Source: three-view drawing plus pictorial views. Frame: mm from the lowest corner of the part. Give positions to 0.01 mm unless a question says otherwise; leave off trailing zeros. Loops run counter-clockwise (first coordinate to the right, second up) from the corner with the lowest first, then second, coordinate; pieces in that order, holes last. Notation, with made-up numbers: M -15.75,61.5 L -1.75,61.5 A11 ccw -1.75,82.5 Z; hole C 57.25,-16.5 d9. An arc over 180 degrees is marked long. Answer as a JSON object with one key per item and string values. Group by question number.
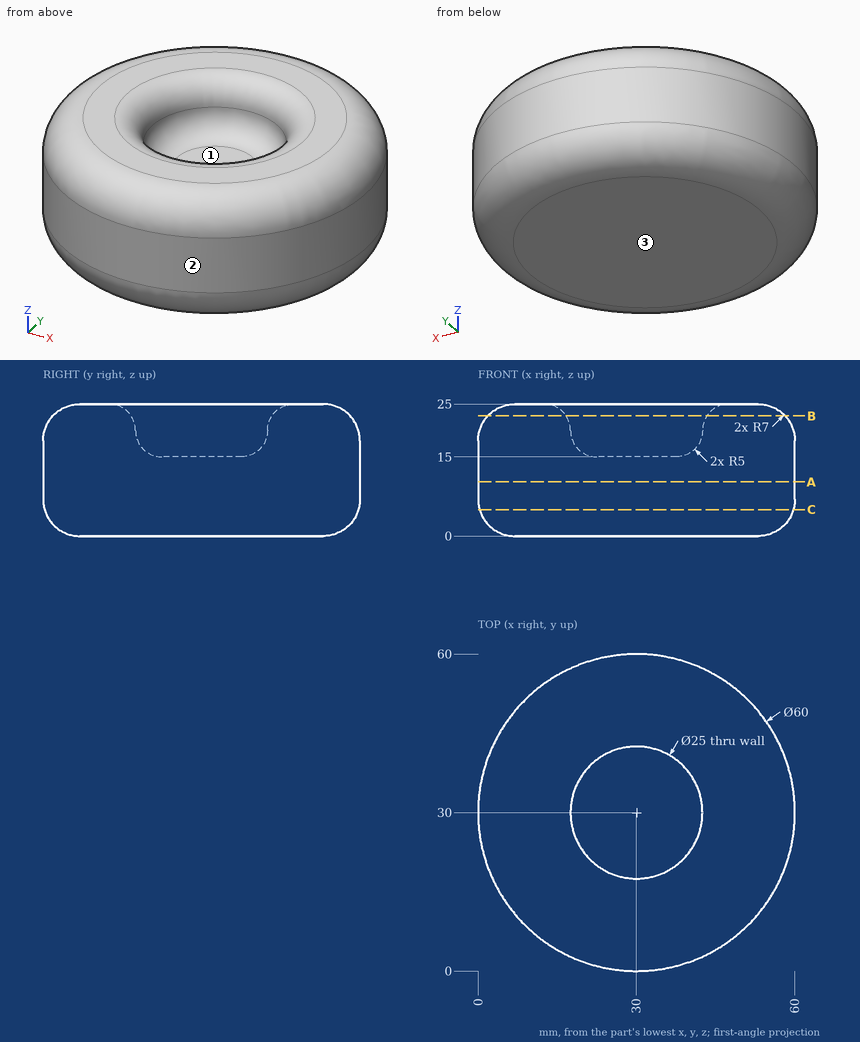
1. Material intervals for L1, parallel to X at y = 31.5, z = 20.75; L2, parallel to Z at x = 16, y = 48.5; L3, parallel to Y at x = 30, z = 20, sorted ascending.
2. Mould query, pull axis X, two halves, no side actions, for the marked faces 1, 2 and 3. Classes: pulls with the +X half, pulls with the -X half, needs draft (parallel to the pull), parting line crosses it, or undercut.
3. Section C-C (z = 5). Output: boundary loops of the cut face in (x, y).
4. Section B-B (z = 22.75). Output: boundary loops of the cut face in (x, y), then the cut area to 3 significant figures.
5. Section A-A (z = 10.25). Output: boundary loops of the cut face in (x, y), then the cut area to 3 significant figures.
6. First-contact query: P1, Ø2, axis at x = 15.5, z = 21.5, coming from the -Y side; P2, Ø6, axis at x = 48.5, z = 17, coming from the -Y side; P3, Ø16.5, axis at x = 26.5, y = 30.5, coming from the +Z side. Flat tips, straight axial feed; report the tip coordinate or a pass-through.
Geometry results:
{
 "1": {"L1": "0.6 to 17.53, 42.47 to 59.4", "L2": "0 to 25", "L3": "0.29 to 17.5, 42.5 to 59.71"},
 "2": {"face 1": "undercut", "face 2": "parting line crosses it", "face 3": "needs draft"},
 "3": {"outline": "C 30,30 d59.42"},
 "4": {"outline": "C 30,30 d56.28; hole C 30,30 d26.65", "area": "1,930 mm2"},
 "5": {"outline": "C 30,30 d60", "area": "2,830 mm2"},
 "6": {"P1": "y = 4.01", "P2": "y = 4.31", "P3": "z = 17.42"}
}
